from build123d import *

# Parameters (mm, degrees)
SKETCH1_W                        = 84
SKETCH1_H                        = 84
BOSS_EXTRUDE1_DEPTH              = 20
M3_CLEARANCE_HOLE1_D             = 3.4
M3_CLEARANCE_HOLE1_CSINK_D       = 3.45
M3_CLEARANCE_HOLE1_CSINK_ANGLE   = 90
BOSS_EXTRUDE2_DEPTH              = 65
SKETCH7_W                        = 84
SKETCH7_H                        = 45
BOSS_EXTRUDE3_DEPTH              = 10
M2_5_CLEARANCE_HOLE2_D           = 2.9
M2_5_CLEARANCE_HOLE2_DEPTH       = 10
M2_5_CLEARANCE_HOLE2_CSINK_D     = 2.95
M2_5_CLEARANCE_HOLE2_CSINK_ANGLE = 90
M2_5_CLEARANCE_HOLE2_TIP         = 0.871247898
SKETCH16_W                       = 30
SKETCH16_H                       = 55
CUT_EXTRUDE2_DEPTH               = 50
CUT_EXTRUDE3_DEPTH               = 124.794184031
CUT_EXTRUDE4_DEPTH               = 230
SKETCH19_W                       = 16
SKETCH19_H                       = 65
CUT_EXTRUDE5_DEPTH               = 230


with BuildPart() as part:
    # Sketch1 → Boss-Extrude1 (new body)
    with BuildSketch(Plane(origin=(0, 0, 0), x_dir=(1, 0, 0), z_dir=(0, 1, 0))):
        Rectangle(SKETCH1_W, SKETCH1_H)
    extrude(amount=BOSS_EXTRUDE1_DEPTH)

    # M3 Clearance Hole1 (through all)
    with Locations(Plane(origin=(0, 20, 0), x_dir=(1, 0, 0), z_dir=(0, 1, 0))):
        with Locations((-34, 34), (34, 34), (34, -34), (-34, -34)):
            CounterSinkHole(M3_CLEARANCE_HOLE1_D / 2, M3_CLEARANCE_HOLE1_CSINK_D / 2, counter_sink_angle=M3_CLEARANCE_HOLE1_CSINK_ANGLE)

    # Sketch5 → Boss-Extrude2 (add)
    with BuildSketch(Plane(origin=(0, 20, 0), x_dir=(1, 0, 0), z_dir=(0, 1, 0))):
        Polygon((-42, 4), (-26, 4), (-26, 42), (26, 42), (26, 4), (42, 4), (42, -72), (-42, -72), align=None)
    extrude(amount=BOSS_EXTRUDE2_DEPTH)

    # Sketch7 → Boss-Extrude3 (add)
    with BuildSketch(Plane(origin=(0, 85, 0), x_dir=(1, 0, 0), z_dir=(0, 1, 0))):
        with Locations((0, -19.5)):
            Rectangle(SKETCH7_W, SKETCH7_H)
    extrude(amount=-BOSS_EXTRUDE3_DEPTH)

    # M2.5 Clearance Hole2
    with Locations(Plane(origin=(0, 85, 0), x_dir=(1, 0, 0), z_dir=(0, 1, 0))):
        with Locations((-18, -58), (18, -58)):
            CounterSinkHole(M2_5_CLEARANCE_HOLE2_D / 2, M2_5_CLEARANCE_HOLE2_CSINK_D / 2, depth=M2_5_CLEARANCE_HOLE2_DEPTH, counter_sink_angle=M2_5_CLEARANCE_HOLE2_CSINK_ANGLE)
            with Locations((0, 0, -(M2_5_CLEARANCE_HOLE2_DEPTH + M2_5_CLEARANCE_HOLE2_TIP / 2))):  # 118° drill point
                Cone(0, M2_5_CLEARANCE_HOLE2_D / 2, M2_5_CLEARANCE_HOLE2_TIP, mode=Mode.SUBTRACT)

    # Sketch16 → Cut-Extrude2 (cut)
    with BuildSketch(Plane.XY.offset(72)):
        with Locations((27, 47.5)):
            Rectangle(SKETCH16_W, SKETCH16_H)
        with Locations((-27, 47.5)):
            Rectangle(SKETCH16_W, SKETCH16_H)
    extrude(amount=-CUT_EXTRUDE2_DEPTH, mode=Mode.SUBTRACT)

    # Sketch17 → Cut-Extrude3 (cut, through all)
    with BuildSketch(Plane(origin=(12, 0, 0), x_dir=(0, 0, -1), z_dir=(1, 0, 0))):
        Polygon((-42, 20), (-72, 75), (-72, 20), align=None)
    extrude(amount=-CUT_EXTRUDE3_DEPTH, mode=Mode.SUBTRACT)

    # Sketch18 → Cut-Extrude4 (cut)
    with BuildSketch(Plane(origin=(26, 0, 0), x_dir=(0, 0, -1), z_dir=(1, 0, 0))):
        Polygon((4, 85), (42, 20), (42, 85), align=None)
    extrude(amount=-CUT_EXTRUDE4_DEPTH, mode=Mode.SUBTRACT)

    # Sketch19 → Cut-Extrude5 (cut)
    with BuildSketch(Plane(origin=(0, 0, -4), x_dir=(-1, 0, 0), z_dir=(0, 0, -1))):
        with Locations((-34, 52.5)):
            Rectangle(SKETCH19_W, SKETCH19_H)
        with Locations((34, 52.5)):
            Rectangle(SKETCH19_W, SKETCH19_H)
    extrude(amount=-CUT_EXTRUDE5_DEPTH, mode=Mode.SUBTRACT)


solid = part.part
Model file for the job. Use its own axes, mm. A direction names the side the tool comes from. Give positions to 0.01 mm unless a question says otherwise; leave off trailing zeros. Write each loop counter-clockwise with the first axis right and the second up, starting at its lowest first coordinate (ties: lowest second). Pieces come first, ordered by that corner, then holes. Notation, with made-up numbers: (0.5, 23) - (11.5, 23) arc R24 ccw to (11.5, 53) - close; hole circle Ø7 at (-25.5, 52.25). An arc over 180 degrees is marked (long way). Answer as CSV lines item,"result".
1. 3-axis set-ups, long thin cutter, end or side, ignore diameter. For faces 4 (the face through (26, 52, 2)), 5 (the face through (-31, 20, 9)), 6 (the face through (-26, 52, 3)): which of +Z, -Z, +X, -X, +Y, -Y reach the whole face in a straight line?
Responses:
face 4,"+Z, -Z, +X, +Y"
face 5,"+Z, -X"
face 6,"+Z, -Z, -X, +Y"
2. Band-saw the part on D-D (z = 12). Write the cut outline in (x, y).
Responses:
outline,"(-42, 0) - (42, 0) - (42, 20) - (26, 20) - (26, 85) - (-26, 85) - (-26, 20) - (-42, 20) - close"
3. Band-saw the part on B-B (z = 34). Write the cut outline in (x, y) (3 decimals).
Responses:
outline,"(-42, 0) - (-35.7, 0) - (-35.7, 19.975) - (-35.725, 20) - (-42, 20) - close; (-32.3, 0) - (32.3, 0) - (32.3, 19.975) - (32.275, 20) - (12, 20) - (12, 75) - (26, 75) - (26, 85) - (-26, 85) - (-26, 75) - (-12, 75) - (-12, 20) - (-32.275, 20) - (-32.3, 19.975) - close; (35.7, 0) - (42, 0) - (42, 20) - (35.725, 20) - (35.7, 19.975) - close"
4. Band-saw the part on A-A (x = -34). Write the cut outline in (y, z) (3 decimals).
Responses:
outline,"(0, -42) - (20, -42) - (20, -35.725) - (19.975, -35.7) - (0, -35.7) - close; (0, -32.3) - (19.975, -32.3) - (20, -32.275) - (20, 32.275) - (19.975, 32.3) - (0, 32.3) - close; (0, 35.7) - (19.975, 35.7) - (20, 35.725) - (20, 42) - (0, 42) - close"
5. Pin check, flat tips, straight feed: pin 1 (2 mm diameter, centred on y = 35, z = 6.5, fed in from +X); pin 2 (10 mm diameter, centred on x = 9, y = 10.5, fed in from +Z); pin 3 (19.5 mm diameter, centred on y = 67, z = 18.5, fed in from -X). Stop position of each tip, or through.
Responses:
pin 1,"stops at x = 26"
pin 2,"stops at z = 42"
pin 3,"stops at x = -26"
6. Drill centre lines: L1, parallel to X at y = 5, z = 34; L2, parallel to X at y = 23, z = -4. Where is each one in solid material? Low to high. Write a range as [from, to].
Responses:
L1,"x = [-42, -35.7], [-32.3, 32.3], [35.7, 42]"
L2,"x = [-26, 26]"
7. Band-saw the part on C-C (x = -18). Write the cut outline in (y, z) (3 decimals).
Responses:
outline,"(0, -42) - (20, -42) - (85, -4) - (85, 56.525) - (84.975, 56.55) - (75, 56.55) - (75, 22) - (20, 22) - (20, 42) - (0, 42) - close; (75, 59.45) - (84.975, 59.45) - (85, 59.475) - (85, 72) - (75, 72) - close"
8. Two-plate mould, pull along Z, no slides. Class faces 1 (the face through (19, 48, 22)), 2 (the face through (17.331, 79.918, 59.286)), 3 (the face through (-1, 0, -1)): +Z half, -Z half, draft (parallel to the pull), parting line (faces both ways), or undercut.
Responses:
face 1,"+Z half"
face 2,"undercut"
face 3,"draft"
